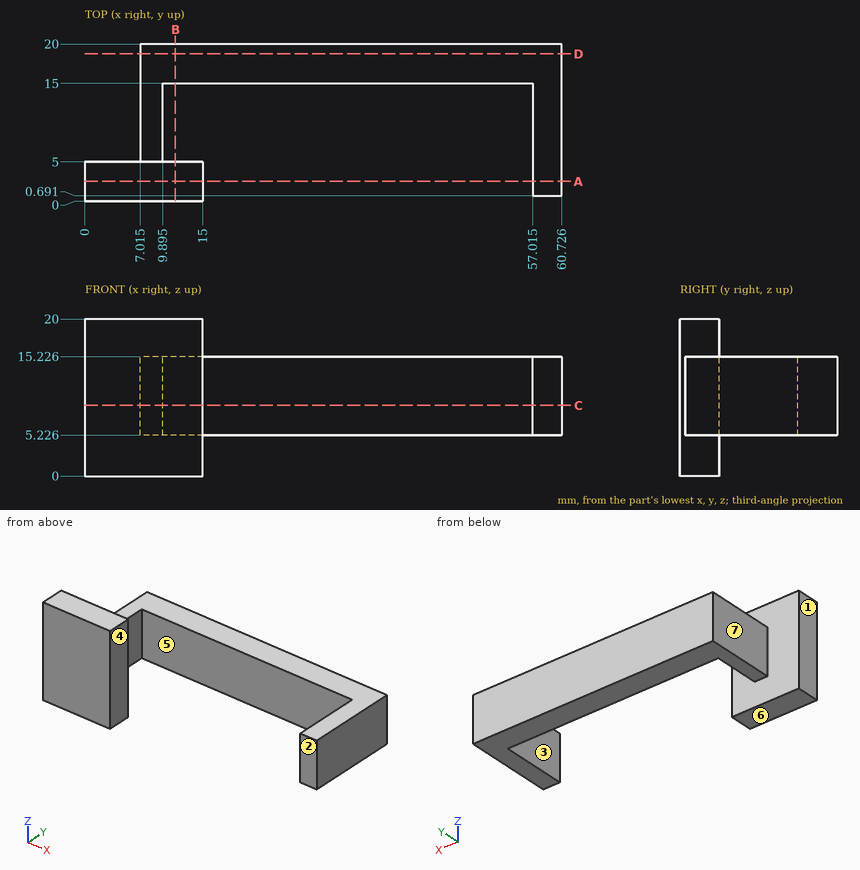
Study the drawing (mm; zero at the part's minimum x, y, z) and answer. A direction names the side the tool comes from. Give positions to 0.01 mm unless a question says otherwise; leave off trailing zeros. Loops run counter-clockwise (first coordinate to the right, second up) from the corner with the lowest first, then second, coordinate; pieces in that order, holes last. Notation, with made-up numbers: (32, 63.25) - (36, 63.25) arc R22 cw to (36, 78.25) - close; hole circle Ø7 at (-39.5, -29). An arc over 180 degrees is marked (long way). Return JSON: item names as keys, results as strings. Group by question number.
1. Find section A-A (y = 2.5). Write down the section's boundary in (x, z) (1 decimal).
2. Find section C-C (z = 9). Write down the section's boundary in (x, y) (1 decimal).
3. Given pin 1 Ø5 at (y, z) = (8, 12.5) entering from -X (1 decimal); pin 2 Ø3 at (x, z) = (58.5, 12.5) entering from -Y; pin 3 Ø11 at (x, z) = (33.5, 9.5) entering from -Y, each flat-ended and moving along its own axis, determine where each tip first touches the part or whether it passes through.
4. Find section D-D (y = 18.75). Write down the section's boundary in (x, z) (1 decimal).
5. Straight lines are drawn through the part: line 1 (X direction, y = 4, z = 8.5) (1 decimal); line 2 (X direction, y = 12.75, z = 7.25) (1 decimal); line 3 (X direction, y = 16.25, z = 13.5) (1 decimal). For each, find the intervals that lie inside material, in ascending order. Write a range as [from, to].
6. Determine the mould class of the marked faces 4, 5, 6 and 7 for opening direction X: pulls with the +X half, pulls with the -X half, needs draft (parallel to the pull), parting line crosses it, or undercut.
7. Which of the six approach directions +Z, -Z, +X, -X, +Y, -Y give full straight-line access (tool end or side, diameter ignored) to the marked faces 1, 2 and 3?
8. Find section B-B (x = 11.5). Write down the section's boundary in (y, z).
Verdict:
{
 "1": {"outline": "(0, 0) - (15, 0) - (15, 20) - (0, 20) - close; (57, 5.2) - (60.7, 5.2) - (60.7, 15.2) - (57, 15.2) - close"},
 "2": {"outline": "(0, 0) - (15, 0) - (15, 5) - (9.9, 5) - (9.9, 15) - (57, 15) - (57, 0.7) - (60.7, 0.7) - (60.7, 20) - (7, 20) - (7, 5) - (0, 5) - close"},
 "3": {"pin 1": "stops at x = 7", "pin 2": "stops at y = 0.69", "pin 3": "stops at y = 15"},
 "4": {"outline": "(7, 5.2) - (60.7, 5.2) - (60.7, 15.2) - (7, 15.2) - close"},
 "5": {"line 1": "x = [0, 15], [57, 60.7]", "line 2": "x = [7, 9.9], [57, 60.7]", "line 3": "x = [7, 60.7]"},
 "6": {"face 4": "undercut", "face 5": "undercut", "face 6": "needs draft", "face 7": "pulls with the -X half"},
 "7": {"face 1": "+Z, -Z, -X, +Y, -Y", "face 2": "+Z, -Z, +X, -Y", "face 3": "+Z, -Z, -Y"},
 "8": {"outline": "(0, 0) - (5, 0) - (5, 20) - (0, 20) - close; (15, 5.23) - (20, 5.23) - (20, 15.23) - (15, 15.23) - close"}
}
